```python
from build123d import *

# Parameters (mm, degrees)
F2_DEPTH    = 76
F3_R        = 12.5
F4_DEPTH    = 127.1
F6_DEPTH    = 53.4
F7_T1_DEPTH = 208.7228714275
F8_W        = 11
F8_H        = 54
F9_DEPTH    = 52
F10_W       = 11
F10_H       = 54
F11_DEPTH   = 52
F13_DEPTH   = 67.9
F14_W       = 50
F14_H       = 38
F15_DEPTH   = 79.6


# Not quite as in the source:
# - a fillet or chamfer that OpenCascade refuses, or shapes differently, is made with other operations: its cross-section is extruded or revolved along the edge and cut away or added


with BuildPart() as f2:
    # F1 (on Right) → F2 (new body)
    with BuildSketch(Plane.YZ):
        Polygon((-74.8220309615, 18), (-74.8220309615, 0), (45.1779690385, 0), (45.1779690385, 72), (-18.8220309615, 72), (-18.8220309615, 18), align=None)
    extrude(amount=F2_DEPTH)

    # F3 (on face) → F4 (cut)
    with BuildSketch(Plane.YZ.offset(76)):
        with Locations((13.1779690385, 36)):
            Circle(F3_R)
    extrude(amount=-F4_DEPTH, mode=Mode.SUBTRACT)

    # F5 (on face) → F6 (cut)
    with BuildSketch(Plane.XY.offset(72)):
        Polygon((13, 32.1779690385), (13, 13.1779690385), (13, -5.8220309615), (28.5150296986, -5.8220309615), (63, -5.8220309615), (63, 16.2556339055), (63, 32.1779690385), (35.4323200881, 32.1779690385), align=None)
    extrude(amount=-F6_DEPTH, mode=Mode.SUBTRACT)

    # F7: fillet of radius 38.1445742855 on 2 edges, made by hand

    # F7_s2 → F7_t1 (cut)
    with BuildSketch(Plane.XY.offset(-95.3614357137)):
        with BuildLine():
            ThreePointArc((38.1445742855, -74.8220309615), (11.1722871427, -63.6497438188), (0, -36.677456676))
            Line((0, -36.677456676), (0, -74.8220309615))
            Line((0, -74.8220309615), (38.1445742855, -74.8220309615))
        make_face()
        with BuildLine():
            ThreePointArc((37.8554257145, -74.8220309615), (64.8277128573, -63.6497438188), (76, -36.677456676))
            Line((76, -36.677456676), (76, -74.8220309615))
            Line((76, -74.8220309615), (37.8554257145, -74.8220309615))
        make_face()
    extrude(amount=F7_T1_DEPTH, mode=Mode.SUBTRACT)

    # F8 (on face) → F9 (join)
    with BuildSketch(Plane.XZ.offset(18.8220309615)):
        with Locations((32.5, 45)):
            Rectangle(F8_W, F8_H)
    extrude(amount=F9_DEPTH)

    # F10 (on face) → F11 (join)
    with BuildSketch(Plane.XZ.offset(18.8220309615)):
        with Locations((43.5, 45)):
            Rectangle(F10_W, F10_H)
    extrude(amount=F11_DEPTH)

    # F12 (on face) → F13 (cut)
    with BuildSketch(Plane.YZ.offset(49)):
        Polygon((-70.8220309615, 72), (-70.8220309615, 18), (-18.8220309615, 72), align=None)
    extrude(amount=-F13_DEPTH, mode=Mode.SUBTRACT)

    # F14 (on face) → F15 (cut)
    with BuildSketch(Plane.XY.offset(18.6)):
        with Locations((38, 13.1779690385)):
            Rectangle(F14_W, F14_H)
    extrude(amount=-F15_DEPTH, mode=Mode.SUBTRACT)


solid = f2.part
```
Could you check a few things on this model? Use its own coordinates, in mm. A direction names the side the tool comes from. Round coordinates to 2 decimals unless told otherwise and drop trailing zeros. Loops run counter-clockwise (first coordinate to the right, second up) from the corner with the lowest first, then second, coordinate; pieces in that order, holes last. Notation, with made-up numbers: (-39.75, 6.5) - (-23.75, 6.5) arc R14 cw to (-23.75, 31.5) - close; hole circle Ø9 at (-38, 27.5). An arc over 180 degrees is marked (long way). Answer in a Markdown table with one row per item. Add a question column.
(1) If we mould it in two halves opening along Z, with no side actions, what happens to faces 1 (the face through (6.59, 3.26, 28.39)), 2 (the face through (37, -8, 72)), 3 (the face through (69.59, 3.26, 28.39)), 4 (the face through (13, 26, 37))? For each: pulls with the +Z half, pulls with the -Z half, needs draft (parallel to the pull), parting line crosses it, or undercut.
(2) I need wall thicknesses on line 1 along Y through (x, z) = (50.5, 33); line 2 along X through (y, z) = (31.5, 20.5); line 3 along X through (y, z) = (-29, 60). Which ranges of each line are inside material? Lowest first, please.
(3) I'm going to push flat-ended pins straight in: pin 1 (1 mm diameter, centred on y = -55.5, z = 32, fed in from -X); pin 2 (8 mm diameter, centred on x = 9.5, y = -57.5, fed in from +Z); pin 3 (4 mm diameter, centred on x = 43, y = -34, fed in from +Z). Where does each tip first touch, or does it pass through?
(4) For faces 5 (the face through (38, 32.178, 37)), 6 (the face through (54, -40, 18)), 7 (the face through (62, -18.822, 45)), 8 (the face through (27, -39, 39)), which set-ups out of +Z, -Z, +X, -X, +Y, -Y let a thin tool reach every point of the face, with its end or its side?
(5) If we section it at D-D (y = 11): Please give me the cut outline in (x, z).
(6) If we section it at B-B (x = 47.5): Please give me the cut outline in (y, z).
(7) If we section it at C-C (z = 34): Please give me the cut outline in (x, y), plus the area to 3 significant figures.
(8) If we section it at A-A (z = 12): Please give me the cut outline in (x, y).
Model answer:
| question | item | result |
|---|---|---|
| 1 | face 1 | undercut |
| 1 | face 2 | pulls with the +Z half |
| 1 | face 3 | undercut |
| 1 | face 4 | needs draft |
| 2 | line 1 | y = -18.82 to -5.82, 32.18 to 45.18 |
| 2 | line 2 | x = 0 to 13, 63 to 76 |
| 2 | line 3 | x = 27 to 49 |
| 3 | pin 1 | stops at x = 27 |
| 3 | pin 2 | stops at z = 18 |
| 3 | pin 3 | stops at z = 58.32 |
| 4 | face 5 | +Z, -Z |
| 4 | face 6 | +Z, -Y |
| 4 | face 7 | +Z, +X, -Y |
| 4 | face 8 | +Z, -X, -Y |
| 5 | outline | (0, 0) - (13, 0) - (13, 23.69) - (0, 23.69) - close; (0, 48.31) - (13, 48.31) - (13, 72) - (0, 72) - close; (63, 0) - (76, 0) - (76, 23.69) - (63, 23.69) - close; (63, 48.31) - (76, 48.31) - (76, 72) - (63, 72) - close |
| 6 | outline | (-73.58, 0) - (-5.82, 0) - (-5.82, 72) - (-18.82, 72) - (-70.82, 18) - (-73.58, 18) - close; (32.18, 0) - (45.18, 0) - (45.18, 72) - (32.18, 72) - close |
| 7 | outline | (0, -18.82) - (27, -18.82) - (27, -55.41) - (49, -55.41) - (49, -18.82) - (76, -18.82) - (76, 0.84) - (63, 0.84) - (63, -5.82) - (13, -5.82) - (13, 0.84) - (0, 0.84) - close; (0, 25.52) - (13, 25.52) - (13, 32.18) - (63, 32.18) - (63, 25.52) - (76, 25.52) - (76, 45.18) - (0, 45.18) - close |
| 7 | area | 3,130 mm² |
| 8 | outline | (0, -36.68) arc R38.14 ccw to (38, -74.82) arc R38.14 ccw to (76, -36.68) - (76, 45.18) - (0, 45.18) - close; hole (13, -5.82) - (63, -5.82) - (63, 32.18) - (13, 32.18) - close |
